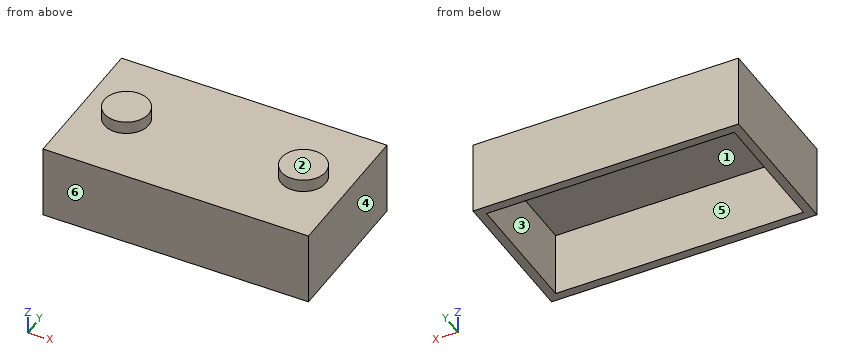
from build123d import *

# Parameters (mm, degrees)
F0_W     = 90
F0_H     = 50
F1_DEPTH = 25
F2_R     = 7.5
F3_DEPTH = 4.3
F4_W     = 84
F4_H     = 44
F5_DEPTH = 22


with BuildPart() as f1:
    # F0 (on Top) → F1 (new body)
    with BuildSketch(Plane.XY):
        Rectangle(F0_W, F0_H)
    extrude(amount=F1_DEPTH)

    # F2 (on face) → F3 (join)
    with BuildSketch(Plane.XY.offset(25)):
        with Locations((30, 0)):
            Circle(F2_R)
        with Locations((-30, 0)):
            Circle(F2_R)
    extrude(amount=F3_DEPTH)

    # F4 (on face) → F5 (cut)
    with BuildSketch(Plane(origin=(0, 0, 0), x_dir=(1, 0, 0), z_dir=(0, 0, -1))):
        Rectangle(F4_W, F4_H)
    extrude(amount=-F5_DEPTH, mode=Mode.SUBTRACT)


solid = f1.part
Work out the finished part from the listing and answer in its coordinate system (mm). Face numbers are marked on the shaded views. A direction names the side the tool comes from. Give positions to 0.01 mm unless a question says otherwise; leave off trailing zeros. Order: outer loops, then holes, each group sorted by start corner. A loop starts at its lowest first (then second) coordinate and runs counter-clockwise, first axis right, second up. Notation, with made-up numbers: (-4.5, 82) -> (7.5, 82) arc R33 ccw to (7.5, 119) -> close; hole circle Ø2 at (-34.75, 0.5). An arc over 180 degrees is marked (long way). One line per item, written item: value.
Item 1: A flat-ended cylindrical pin translates along its axis: P1, Ø8, axis at x = -29.5, y = -9, coming from the -Z side. Find the tip coordinate at first contact, or state that the pin passes through.
Answer sheet:
P1: z = 22
Item 2: A tool of negligible diameter and unlimited length cuts with its end or side. For the marked faces 1 and 2, from which of +Z, -Z, +X, -X, +Y, -Y can it reach the whole face along a straight path? Write none if from no direction.
Answer sheet:
face 1: -Z
face 2: +Z, +X, -X, +Y, -Y
Item 3: Straight lines are drawn through the part: probe 1 along Y at (x, z) = (12, 1); probe 2 along X at (y, z) = (6, 14); probe 3 along Z at (x, y) = (-34, -1). For each, find the intervals that lie inside material, in ascending order.
Answer sheet:
probe 1: -25 to -22, 22 to 25
probe 2: -45 to -42, 42 to 45
probe 3: 22 to 29.3
Item 4: Determine the mould class of the marked faces 3, 4, 5 and 6 for opening direction X: released by +X, released by -X, zero draft, split by the parting line, or undercut.
Answer sheet:
face 3: undercut
face 4: released by +X
face 5: undercut
face 6: zero draft
Item 5: Find section A-A, the plane z = 13.5. Give the vertices of the cut face in (x, y).
Answer sheet:
outline: (-45, -25) -> (45, -25) -> (45, 25) -> (-45, 25) -> close; hole (-42, -22) -> (42, -22) -> (42, 22) -> (-42, 22) -> close
Item 6: Find section B-B, the plane y = 6. Give the vertices of the cut face in (x, z), plus the area to 3 significant figures.
Answer sheet:
outline: (-45, 0) -> (-42, 0) -> (-42, 22) -> (42, 22) -> (42, 0) -> (45, 0) -> (45, 25) -> (34.5, 25) -> (34.5, 29.3) -> (25.5, 29.3) -> (25.5, 25) -> (-25.5, 25) -> (-25.5, 29.3) -> (-34.5, 29.3) -> (-34.5, 25) -> (-45, 25) -> close
area: 479 mm²
Item 7: Find section D-D, the plane y = 12. Give the vertices of the cut face in (x, z), plus the area to 3 significant figures.
Answer sheet:
outline: (-45, 0) -> (-42, 0) -> (-42, 22) -> (42, 22) -> (42, 0) -> (45, 0) -> (45, 25) -> (-45, 25) -> close
area: 402 mm²
Item 8: Find section C-C, the plane x = -30. Give the vertices of the cut face in (y, z).
Answer sheet:
outline: (-25, 0) -> (-22, 0) -> (-22, 22) -> (22, 22) -> (22, 0) -> (25, 0) -> (25, 25) -> (7.5, 25) -> (7.5, 29.3) -> (-7.5, 29.3) -> (-7.5, 25) -> (-25, 25) -> close
